Design review of the part shown in the three views and the two pictorial views. Dimensions are in mm from the part's minimum x, y and z. A direction names the side the tool comes from. Round coordinates to 2 decimals unless told otherwise and drop trailing zeros. Order: outer loops, then holes, each group sorted by start corner. A loop starts at its lowest first (then second) coordinate and runs counter-clockwise, first axis right, second up. Notation, with made-up numbers: (56.5, 19.25) -> (111.5, 19.25) arc R27 ccw to (111.5, 39.25) -> close; hole circle Ø9 at (-20.5, -24.75). An arc over 180 degrees is marked (long way). Put each result on its own line as item: value. Start each with the question number.
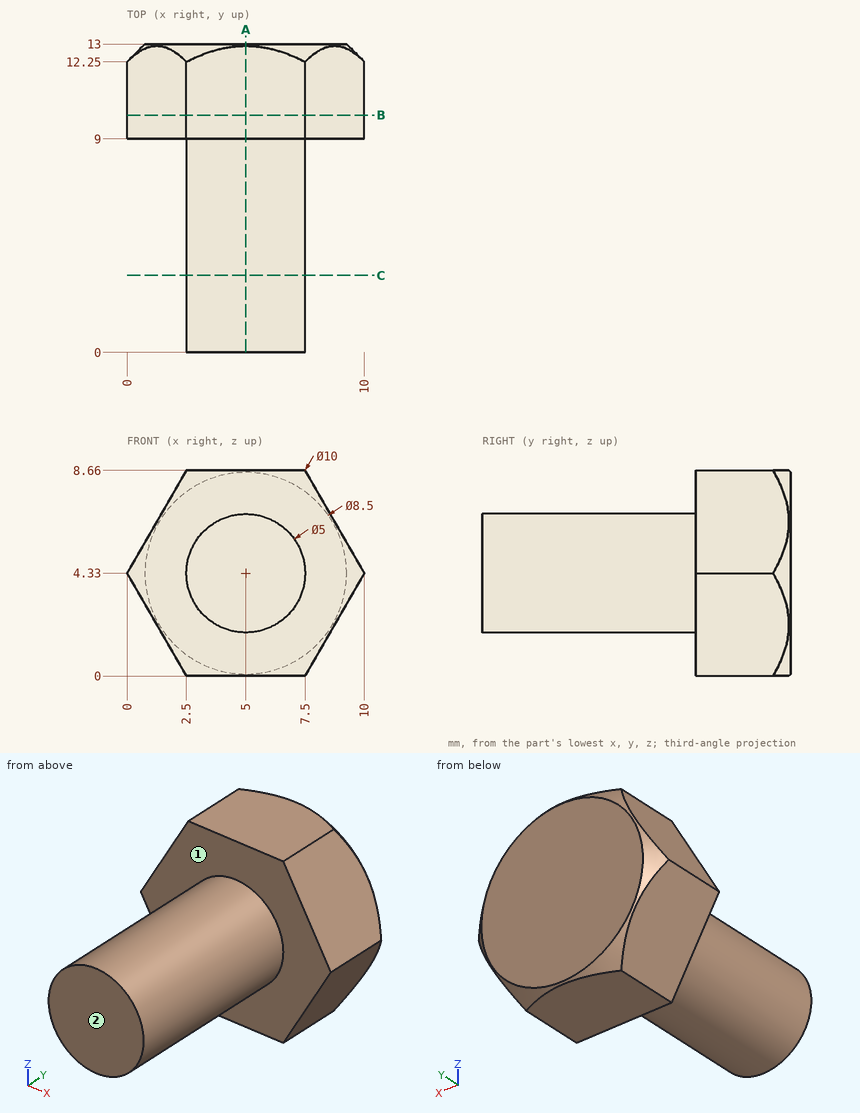
Q1. Wall thickness on probe 1 along Y at (x, z) = (1, 6) (1 decimal); probe 2 along Y at (x, z) = (7.75, 1.25); probe 3 along Z at (x, y) = (5, 0.5): over which ranges is each line inside the solid? List them lowest first. Write a range as [from, to].
Q2. Take a section at C-C on y = 3.25. Give the boundary of the cut face in (x, z), and give its area (3 significant figures).
Q3. Take a section at B-B on y = 10. Give the boundary of the cut face in (x, z).
Q4. Clearance check with flat-ended pins moving along their axes: pin 1 Ø1 at (y, z) = (5, 4) entering from -X; pin 2 Ø3 at (y, z) = (7, 2) entering from -X. State where each tip first meets the part, or that it passes through.
Q5. For the marked faces 1 and 2, list the 3-axis set-ups (+Z, -Z, +X, -X, +Y, -Y) from which the entire face can be reached by the end or side of a thin tool; tool diameter is ignored.
Q6. Take a section at A-A on x = 5. Give the boundary of the cut face in (y, z).
Calculated:
1. probe 1: y = [9, 12.9]
1. probe 2: y = [9, 13]
1. probe 3: z = [1.83, 6.83]
2. outline: circle Ø5 at (5, 4.33)
2. area: 19.6 mm²
3. outline: (0, 4.33) -> (2.5, 0) -> (7.5, 0) -> (10, 4.33) -> (7.5, 8.66) -> (2.5, 8.66) -> close
4. pin 1: stops at x = 2.5
4. pin 2: stops at x = 2.64
5. face 1: -Y
5. face 2: +Z, -Z, +X, -X, -Y
6. outline: (0, 1.83) -> (9, 1.83) -> (9, 0) -> (12.92, 0) -> (13, 0.08) -> (13, 8.58) -> (12.92, 8.66) -> (9, 8.66) -> (9, 6.83) -> (0, 6.83) -> close
